The listing builds one solid part. Answer for the finished solid, in the listing's coordinates (mm). Coordinates: 2 decimals unless noted, no trailing zeros. Write each loop counter-clockwise with the first axis right and the second up, starting at its lowest first coordinate (ties: lowest second). Pieces come first, ordered by that corner, then holes.
(1) Given P1, Ø1.5, axis at y = -19, z = 1.5, coming from the -X side, flat-ended and moving along its own axis, determine where the tip first touches the part or whether it passes through.
(2) The part is cut by section A-A on y = 19. Determine the outline of the cut face in (x, z), plus the area to 3 significant figures.
(3) The part is cut by section B-B on x = 17.5. Determine the outline of the cut face in (y, z).
(4) Straight lines are drawn through the part: line 1 (X direction, y = -14.5, z = 2); line 2 (Y direction, x = 18.5, z = 0.8); line 3 (X direction, y = -0.5, z = 2). For each, find the intervals that lie inside material, in ascending order.
(5) The part is cut by section C-C on z = 1. Determine the outline of the cut face in (x, y).
from build123d import *

# Parameters (mm, degrees)
SKETCH1_W           = 150
SKETCH1_H           = 100
BOSS_EXTRUDE1_DEPTH = 3
CAVITY1_START       = -75
CAVITY1_OUTLINE_W   = 3
CAVITY1_OUTLINE_H   = 3
CAVITY1_DEPTH       = 150
CAVITY1_2_OUTLINE_W = 20
CAVITY1_2_OUTLINE_H = 3
CAVITY1_2_DEPTH     = 3
CAVITY1_START_2     = 72
CAVITY1_3_OUTLINE_W = 20
CAVITY1_3_OUTLINE_H = 3
CAVITY1_3_DEPTH     = 3
SKETCH2_W           = 100
SKETCH2_H           = 70
CUT_EXTRUDE1_DEPTH  = 3


# Read off the part's stored shape, not the designer's step: Cavity1
with BuildPart() as part:
    # Sketch1 → Boss-Extrude1 (new body)
    with BuildSketch(Plane.XY):
        Rectangle(SKETCH1_W, SKETCH1_H)
    extrude(amount=BOSS_EXTRUDE1_DEPTH)

    # Cavity1 outline → Cavity1 (cut)
    with BuildSketch(Plane.YZ.offset(CAVITY1_START)):
        with Locations((48.5, 1.5)):
            Rectangle(CAVITY1_OUTLINE_W, CAVITY1_OUTLINE_H)
        with Locations((-48.5, 1.5)):
            Rectangle(CAVITY1_OUTLINE_W, CAVITY1_OUTLINE_H)
    extrude(amount=CAVITY1_DEPTH, mode=Mode.SUBTRACT)

    # Cavity1 2 outline → Cavity1 2 (cut)
    with BuildSketch(Plane.YZ.offset(CAVITY1_START)):
        with Locations((20, 1.5)):
            Rectangle(CAVITY1_2_OUTLINE_W, CAVITY1_2_OUTLINE_H)
        with Locations((-20, 1.5)):
            Rectangle(CAVITY1_2_OUTLINE_W, CAVITY1_2_OUTLINE_H)
    extrude(amount=CAVITY1_2_DEPTH, mode=Mode.SUBTRACT)

    # Cavity1 3 outline → Cavity1 3 (cut)
    with BuildSketch(Plane.YZ.offset(CAVITY1_START_2)):
        with Locations((20, 1.5)):
            Rectangle(CAVITY1_3_OUTLINE_W, CAVITY1_3_OUTLINE_H)
        with Locations((-20, 1.5)):
            Rectangle(CAVITY1_3_OUTLINE_W, CAVITY1_3_OUTLINE_H)
    extrude(amount=CAVITY1_3_DEPTH, mode=Mode.SUBTRACT)

    # Sketch2 → Cut-Extrude1 (cut)
    with BuildSketch(Plane.XY.offset(3)):
        Rectangle(SKETCH2_W, SKETCH2_H)
    extrude(amount=-CUT_EXTRUDE1_DEPTH, mode=Mode.SUBTRACT)


solid = part.part
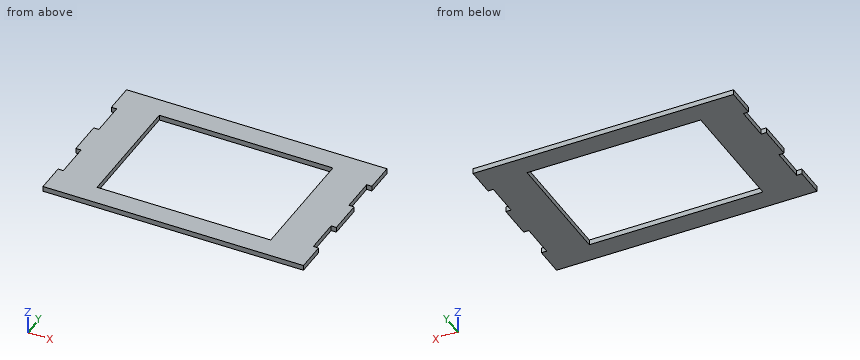
Model answer:
1. P1: stops at x = -72
2. outline: (-72, 0) - (-50, 0) - (-50, 3) - (-72, 3) - close; (50, 0) - (72, 0) - (72, 3) - (50, 3) - close
2. area: 132 mm2
3. outline: (-47, 0) - (-35, 0) - (-35, 3) - (-47, 3) - close; (35, 0) - (47, 0) - (47, 3) - (35, 3) - close
4. line 1: x = -72 to -50, 50 to 72
4. line 2: y = -47 to -35, 35 to 47
4. line 3: x = -75 to -50, 50 to 75
5. outline: (-75, -47) - (75, -47) - (75, -30) - (72, -30) - (72, -10) - (75, -10) - (75, 10) - (72, 10) - (72, 30) - (75, 30) - (75, 47) - (-75, 47) - (-75, 30) - (-72, 30) - (-72, 10) - (-75, 10) - (-75, -10) - (-72, -10) - (-72, -30) - (-75, -30) - close; hole (-50, -35) - (50, -35) - (50, 35) - (-50, 35) - close
